Can you work these out from the model? Positions are in its coordinate system, mm. A direction names the side the tool comes from. Coordinates: 2 decimals unless noted, no trailing zeros. Loops run counter-clockwise (first coordinate to the right, second up) from the corner with the lowest first, then second, coordinate; pieces in that order, holes last.
```python
from build123d import *

# Parameters (mm, degrees)
F0_W     = 9.2
F0_H     = 39.5
F0_W_2   = 2.8
F0_H_2   = 16
F1_DEPTH = 1.45
F2_DEPTH = 17
F3_R     = 7.99999
F4_R     = 2.5
F5_DEPTH = 25
F6_R     = 1


# Not quite as in the source:
# - a fillet or chamfer is up to 0.001 mm smaller than in the source, because OpenCascade refuses the exact size


with BuildPart() as f1:
    # F0 (on Top) → F1 (new body)
    with BuildSketch(Plane.XY):
        with Locations((0.1172406439, 4.75)):
            Rectangle(F0_W, F0_H)
        with Locations((-2.9827593561, 4)):
            Rectangle(F0_W_2, F0_H_2, mode=Mode.SUBTRACT)
        with Locations((3.2172406439, 4)):
            Rectangle(F0_W_2, F0_H_2, mode=Mode.SUBTRACT)
    extrude(amount=F1_DEPTH)

    # F0 (on Top) → F2 (join)
    with BuildSketch(Plane.XY):
        with Locations((-2.9827593561, 4)):
            Rectangle(F0_W_2, F0_H_2)
        with Locations((3.2172406439, 4)):
            Rectangle(F0_W_2, F0_H_2)
    extrude(amount=F2_DEPTH)

    # F3 (radius 8 in the source; OpenCascade refuses exactly that, so slightly less here)
    f3_edges = [f1.edges().sort_by_distance(p)[0] for p in [
        (-2.982759, 12, 17),
        (3.217241, 12, 17),
        (3.217241, -4, 17),
        (-2.982759, -4, 17),
    ]]
    fillet(f3_edges, radius=F3_R)

    # F4 (on face) → F5 (cut)
    with BuildSketch(Plane.YZ.offset(4.6172406439)):
        with Locations((4, 9.6)):
            Circle(F4_R)
    extrude(amount=-F5_DEPTH, mode=Mode.SUBTRACT)

    # F6
    f6_edges = [f1.edges().sort_by_distance(p)[0] for p in [
        (4.717241, 24.5, 0.725),
        (-4.482759, 24.5, 0.725),
        (4.717241, -15, 0.725),
        (-4.482759, -15, 0.725),
    ]]
    fillet(f6_edges, radius=F6_R)


solid = f1.part
```
Item 1: Suppose I cut it at A-A, the plane z = 4.5. Please give me the cut outline in (x, y), plus the area to 3 significant figures.
Results are:
outline: (-4.38, -4) - (-1.58, -4) - (-1.58, 12) - (-4.38, 12) - close; (1.82, -4) - (4.62, -4) - (4.62, 12) - (1.82, 12) - close
area: 89.6 mm2
Item 2: We'd pull the mould along Y, two halves only. Please class faces 1 (the face through (3.237, 6.385, 10.351)), 2 (the face through (-4.383, 6, 7)), 3 (the face through (-2.963, -1.594, 14.719)): +Y half, -Y half, draft (parallel to the pull), parting line (faces both ways), or undercut.
Results are:
face 1: undercut
face 2: draft
face 3: -Y half
Item 3: I'm going to push flat-ended pins straight in: P1, Ø0.8, axis at x = -2.5, z = 3.5, coming from the -Y side; P2, Ø3, axis at x = -0.5, y = 5, coming from the +Z side; P3, Ø2, axis at x = 0, z = 5, coming from the +Y side; P4, Ø5, axis at x = -3.5, z = 5, coming from the +Y side. Where does each tip first touch, or does it pass through?
Results are:
P1: stops at y = -4
P2: stops at z = 17
P3: passes through
P4: stops at y = 12
Item 4: Suppose I cut it at C-C, the plane z = 11.25. Please give me the cut outline in (x, y), plus the area to 3 significant figures.
Results are:
outline: (-4.38, -3.68) - (-1.58, -3.68) - (-1.58, 2.12) - (-4.38, 2.12) - close; (-4.38, 5.88) - (-1.58, 5.88) - (-1.58, 11.68) - (-4.38, 11.68) - close; (1.82, -3.68) - (4.62, -3.68) - (4.62, 2.12) - (1.82, 2.12) - close; (1.82, 5.88) - (4.62, 5.88) - (4.62, 11.68) - (1.82, 11.68) - close
area: 64.9 mm2
Item 5: On a 3-axis mill with a long thin cutter (end or side, diameter ignored), from which of +Z, -Z, +X, -X, +Y, -Y can I reach the whole of each face in a straight line? I mean faces 4 (the face through (3, -4, 5)), 5 (the face through (-3, 12, 5)), 6 (the face through (-1.583, 6, 7)). Say none if no direction works.
Results are:
face 4: +Z, +X, -X, -Y
face 5: +Z, +X, -X, +Y
face 6: +Z, +Y, -Y
Item 6: I need wall thicknesses on line 1 along X through (y, z) = (-2, 4); line 2 along Z through (x, y) = (-2.35, 4); line 3 along Z through (x, y) = (0.5, 2). Which ranges of each line are inside material? Lowest first, please.
Results are:
line 1: x = -4.38 to -1.58, 1.82 to 4.62
line 2: z = 0 to 7.1, 12.1 to 17
line 3: z = 0 to 1.45
Item 7: Suppose I cut it at D-D, the plane y = 18.5. Please give me the cut outline in (x, z), plus the area to 3 significant figures.
Results are:
outline: (-4.48, 0) - (4.72, 0) - (4.72, 1.45) - (-4.48, 1.45) - close
area: 13.3 mm2
